from build123d import *

# Parameters (mm, degrees)
F0_W     = 200
F0_H     = 120
F1_DEPTH = 6.35
F3_SIZE  = 5.08
F4_W     = 56.922462
F4_H     = 8.15711
F5_DEPTH = 1.5875
F6_SIZE  = 1.27
F2_R     = 19.05
F7_DEPTH = 3
F8_W     = 55.5
F8_H     = 2
F9_DEPTH = 2


with BuildPart() as f1:
    # F0 (on Top) → F1 (new body)
    with BuildSketch(Plane.XY):
        with Locations((-100, 60)):
            Rectangle(F0_W, F0_H)
    extrude(amount=F1_DEPTH)

    # F3
    f3_edges = [f1.edges().sort_by_distance(p)[0] for p in [
        (-200, 60, 6.35),
        (-100, 120, 6.35),
        (-100, 0, 6.35),
        (0, 60, 6.35),
    ]]
    chamfer(f3_edges, length=F3_SIZE)

    # F4 (on face) → F5 (join)
    with BuildSketch(Plane.XY.offset(6.35)):
        with Locations((-113.111961, 19.376122)):
            Rectangle(F4_W, F4_H)
    extrude(amount=F5_DEPTH)

    # F6
    f6_edges = [f1.edges().sort_by_distance(p)[0] for p in [
        (-113.111961, 15.297567, 7.9375),
        (-141.573192, 19.376122, 7.9375),
        (-113.111961, 23.454677, 7.9375),
        (-84.65073, 19.376122, 7.9375),
    ]]
    chamfer(f6_edges, length=F6_SIZE)

    # F2 (on face) → F7 (cut)
    with BuildSketch(Plane.XY.offset(6.35)):
        with Locations((-55, 40)):
            Circle(F2_R)
    extrude(amount=-F7_DEPTH, mode=Mode.SUBTRACT)

    # F8 (on face) → F9 (cut)
    with BuildSketch(Plane.XY.offset(6.35)):
        with Locations((-107.8826, 78.554325)):
            Rectangle(F8_W, F8_H)
        with Locations((-107.8826, 61.554325)):
            Rectangle(F8_W, F8_H)
    extrude(amount=-F9_DEPTH, mode=Mode.SUBTRACT)


solid = f1.part
Model file for the job. Use its own axes, mm. A direction names the side the tool comes from. Give positions to 0.01 mm unless a question says otherwise; leave off trailing zeros. Order: outer loops, then holes, each group sorted by start corner. A loop starts at its lowest first (then second) coordinate and runs counter-clockwise, first axis right, second up. Notation, with made-up numbers: M 18,43.25 L 61,43.25 A7 ccw 61,47.25 Z; hole C -23.5,-2 d8. An arc over 180 degrees is marked long. Write item = value, one per line.
Q1. Tool access for faces 4 (the flat face through (-55, 40, 3.35)), 5 (the flat face through (-101.4, 117.42, 3.85)): list every direction of +Z, -Z, +X, -X, +Y, -Y with a clear straight run to the whole face (end or side of a thin tool).
Derived:
face_4 = +Z
face_5 = +Z, +X, -X, +Y
Q2. Cut at D-D, the plane y = 105.5. List the corners of the cut face in (x, z).
Derived:
outline = M -200,0 L 0,0 L 0,1.27 L -5.08,6.35 L -194.92,6.35 L -200,1.27 Z
Q3. Cut at C-C, the plane x = -165. List the corners of the cut face in (y, z), then the cut area to 3 significant figures.
Derived:
outline = M 0,0 L 120,0 L 120,1.27 L 114.92,6.35 L 5.08,6.35 L 0,1.27 Z
area = 736 mm2
Q4. Cut at A-A, the plane x = -88. List the corners of the cut face in (y, z).
Derived:
outline = M 0,0 L 120,0 L 120,1.27 L 114.92,6.35 L 79.55,6.35 L 79.55,4.35 L 77.55,4.35 L 77.55,6.35 L 62.55,6.35 L 62.55,4.35 L 60.55,4.35 L 60.55,6.35 L 23.45,6.35 L 23.45,6.67 L 22.18,7.94 L 16.57,7.94 L 15.3,6.67 L 15.3,6.35 L 5.08,6.35 L 0,1.27 Z
Q5. Two-plate mould, pull along X, no slides. Class faces 1 (the flat face through (-197.42, 59.16, 3.85)), 2 (the cylindrical face through (-59.13, 21.403, 4.871)), 3 (the flat face through (-113, 19, 7.938)): pulls with the +X half, pulls with the -X half, needs draft (parallel to the pull), parting line crosses it, or undercut.
Derived:
face_1 = pulls with the -X half
face_2 = undercut
face_3 = needs draft
Q6. Drill centre lines: line 1 (Y direction, x = -117, z = 4.5); line 2 (Y direction, x = -106, z = 5.25); line 3 (Z direction, x = -9, y = 9.5). Where is each one in solid material? Low to high. Write a range as [from, to].
Derived:
line_1 = [3.23, 60.55], [62.55, 77.55], [79.55, 116.77]
line_2 = [3.98, 60.55], [62.55, 77.55], [79.55, 116.02]
line_3 = [0, 6.35]
Q7. Cut at B-B, the plane y = 40. List the corners of the cut face in (x, z).
Derived:
outline = M -200,0 L 0,0 L 0,1.27 L -5.08,6.35 L -35.95,6.35 L -35.95,3.35 L -74.05,3.35 L -74.05,6.35 L -194.92,6.35 L -200,1.27 Z
Q8. Flat gauge pins, fed straight in: pin 1 (1 mm diameter, centred on y = 61.5, z = 5.5, fed in from +X); pin 2 (1 mm diameter, centred on y = 61.5, z = 5, fed in from -X); pin 3 (2 mm diameter, centred on x = -119, z = 5.5, fed in from +Y). Where does each tip first touch, or does it go through?
Derived:
pin_1 = -3.73
pin_2 = -196.77
pin_3 = 116.77
